Verification items for this drawing (mm, ordinates from the low corner). A direction names the side the tool comes from. Round coordinates to 2 decimals unless told otherwise and drop trailing zeros. Order: outer loops, then holes, each group sorted by start corner. A loop starts at its lowest first (then second) coordinate and runs counter-clockwise, first axis right, second up. Notation, with made-up numbers: M -9.75,26.25 L 5.25,26.25 A26 cw 5.25,46.25 Z; hole C 74.25,18 d9. An arc over 180 degrees is marked long. Return JSON: item names as keys, results as strings. Group by question number.
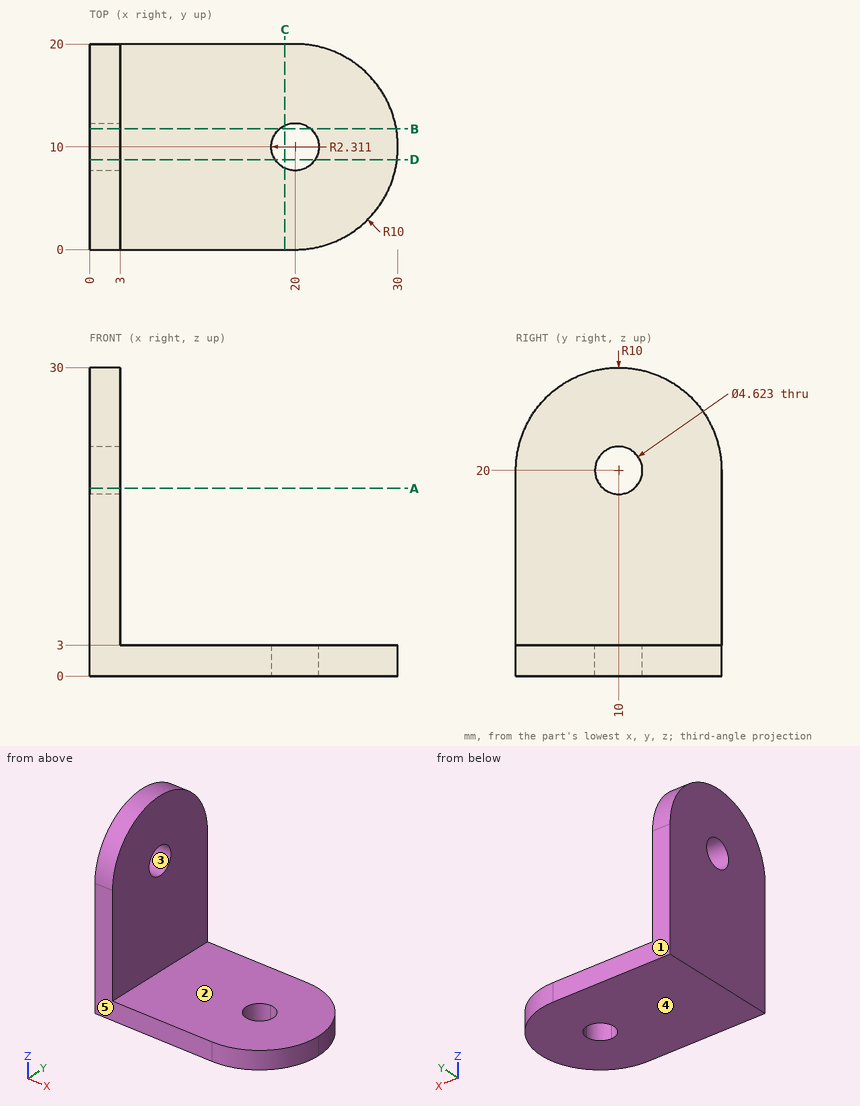
1. Cross-section at D-D (y = 8.75). Enter the section's corners in (x, z) (1 decimal), plus the area to 3 significant figures.
2. Cross-section at B-B (y = 11.75). Enter the section's corners in (x, z) (1 decimal).
3. Access from +Z, -Z, +X, -X, +Y, -Y to the whole of each face (thin tool, end or side, straight path). Record for the marked faces 1 and 2.
4. Thickness scan on line 1 along Z through (x, y) = (2.4, 10); line 2 along X through (y, z) = (4, 22). Record the ranges inside material, lowest first. Write a range as from..to.
5. Draft check along Y on the marked faces 3, 4 and 5. Enter one of: +Y half, -Y half, draft (parallel to the pull), parting line (faces both ways), or undercut.
6. Go/stop test with flat-tipped pins: pin 1 (12 mm diameter, centred on x = 3.5, y = 9.5, fed in from -Z); pin 2 (10 mm diameter, centred on y = 6, z = 20.5, fed in from +X). Record where each tip stops, or that it passes through.
7. Cross-section at A-A (z = 18.25). Enter the section's corners in (x, y).
8. Cross-section at C-C (x = 19). Enter the section's corners in (y, z).
Computed:
{
 "1": {"outline": "M 0,0 L 18.1,0 L 18.1,3 L 3,3 L 3,18.1 L 0,18.1 Z; M 0,21.9 L 3,21.9 L 3,29.9 L 0,29.9 Z; M 21.9,0 L 29.9,0 L 29.9,3 L 21.9,3 Z", "area": "147 mm²"},
 "2": {"outline": "M 0,0 L 18.5,0 L 18.5,3 L 3,3 L 3,18.5 L 0,18.5 Z; M 0,21.5 L 3,21.5 L 3,29.8 L 0,29.8 Z; M 21.5,0 L 29.8,0 L 29.8,3 L 21.5,3 Z"},
 "3": {"face 1": "+Z, -Z, +X, -X, +Y", "face 2": "+Z, +X, +Y, -Y"},
 "4": {"line 1": "z = 0..17.69, 22.31..30", "line 2": "x = 0..3"},
 "5": {"face 3": "undercut", "face 4": "draft", "face 5": "-Y half"},
 "6": {"pin 1": "stops at z = 0", "pin 2": "stops at x = 3"},
 "7": {"outline": "M 0,0 L 3,0 L 3,8.49 L 0,8.49 Z; M 0,11.51 L 3,11.51 L 3,20 L 0,20 Z"},
 "8": {"outline": "M 0,0 L 7.92,0 L 7.92,3 L 0,3 Z; M 12.08,0 L 20,0 L 20,3 L 12.08,3 Z"}
}
